Answer from the drawing. Dimensions are ordinates in mm from the lowest x, y and z of the part. Round coordinates to 2 decimals unless told otherwise and drop trailing zeros. Loops run counter-clockwise (first coordinate to the right, second up) from the corner with the lowest first, then second, coordinate; pieces in that order, holes last. Notation, with made-up numbers: (38, -38) - (83, -38) arc R33 cw to (83, -8) - close; hole circle Ø6 at (47.5, -38.5). An arc over 180 degrees is marked (long way). Answer as CSV lines item,"result". Start each with the question number.
Q1. Section A-A on y = 3.75 is taken. Write down the section's boundary in (x, z).
Q2. Straight lines are drawn through the part: L1, parallel to X at y = 1.95, z = 3.25; L2, parallel to X at y = 1.7, z = 25.5; L3, parallel to Z at x = 68, y = 1.1. For each, find the intervals that lie inside material, in ascending order. Write a range as [from, to].
Q3. Each of these flat-tipped pins is pushed along its axis until it touches: pin 1 Ø2.5 at (x, z) = (68, 3.25) entering from -Y; pin 2 Ø1.2 at (x, z) = (68, 47.25) entering from -Y. Where does it stop, or does it pass through?
Q4. Section C-C on z = 12.5 is taken. Write down the section's boundary in (x, y), then the cut area to 3 significant figures.
Q5. The mould has two halves that part along X. Classify the marked faces 1 and 2: +X half, -X half, draft (parallel to the pull), parting line (faces both ways), or undercut.
Q6. Section B-B on x = 32 is taken. Write down the section's boundary in (y, z).
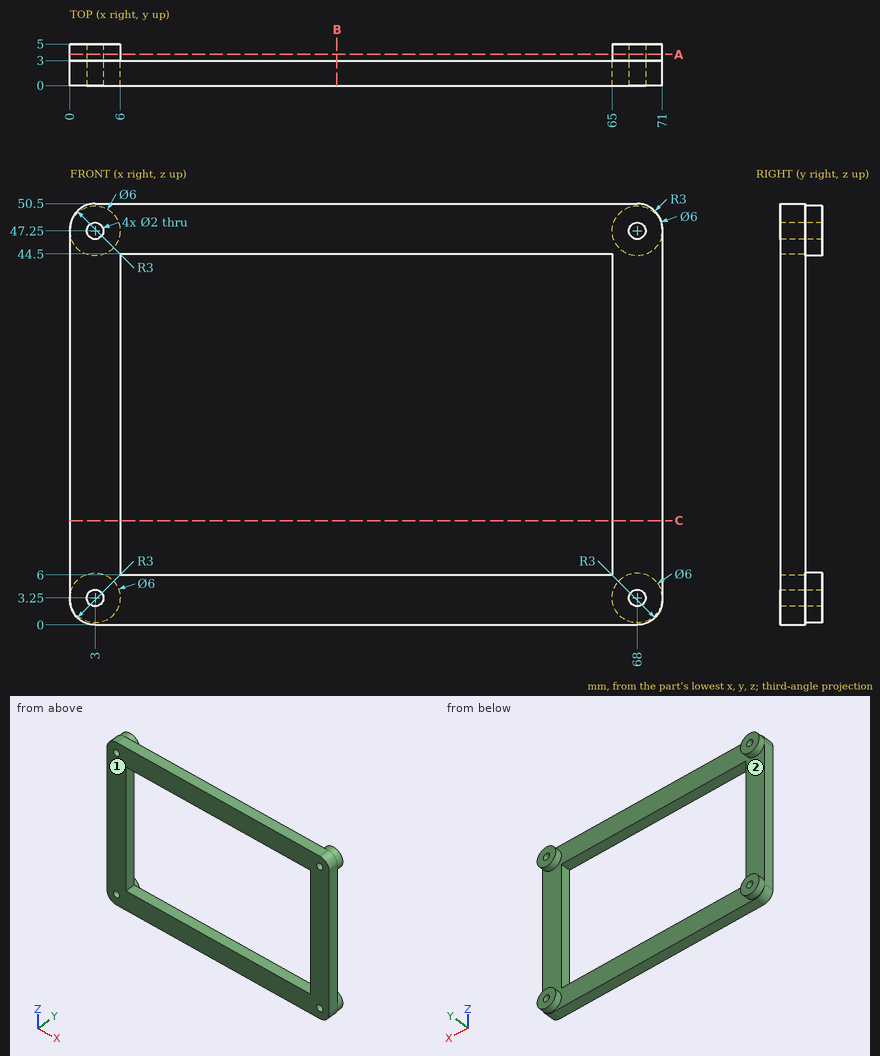
Findings:
1,outline,"circle Ø6 at (3, 3.25); circle Ø6 at (3, 47.25); circle Ø6 at (68, 3.25); circle Ø6 at (68, 47.25); hole circle Ø2 at (3, 3.25); hole circle Ø2 at (3, 47.25); hole circle Ø2 at (68, 3.25); hole circle Ø2 at (68, 47.25)"
2,L1,"x = [0, 2], [4, 67], [69, 71]"
2,L2,"x = [0, 6], [65, 71]"
2,L3,"z = [0, 2.25], [4.25, 46.25], [48.25, 50.5]"
3,pin 1,"stops at y = 0"
3,pin 2,"passes through"
4,outline,"(0, 0) - (6, 0) - (6, 3) - (0, 3) - close; (65, 0) - (71, 0) - (71, 3) - (65, 3) - close"
4,area,"36.0 mm^2"
5,face 1,"draft"
5,face 2,"undercut"
6,outline,"(0, 0) - (3, 0) - (3, 6) - (0, 6) - close; (0, 44.5) - (3, 44.5) - (3, 50.5) - (0, 50.5) - close"
